Autodesk Inventor part; units mm, degrees
ref_plane "YZ Plane" through (0, 0, 0) normal (1, 0, 0) x (0, 1, 0)
ref_plane "XZ Plane" through (0, 0, 0) normal (0, 1, 0) x (-1, 0, 0)
ref_plane "XY Plane" through (0, 0, 0) normal (0, 0, 1) x (1, 0, 0)
sketch "Skizze1" plane through (0, 0, 0) normal (0, 0, 1) x (1, 0, 0)
  line L0 (46.5, 52.5) -> (-46.5, 52.5)
  line L1 (-46.5, 52.5) -> (-46.5, -52.5)
  line L2 (-46.5, -52.5) -> (46.5, -52.5)
  line L3 (46.5, -52.5) -> (46.5, 52.5)
  circle A0 centre (49, -60.25) radius 5.3
  circle A1 centre (49, -60.25) radius 2
  circle A2 centre (49, 60.25) radius 5.3
  circle A3 centre (49, 60.25) radius 2
  circle A4 centre (-61, 60.25) radius 5.3
  circle A5 centre (-61, 60.25) radius 2
  circle A6 centre (-61, -60.25) radius 5.3
  circle A7 centre (-61, -60.25) radius 2
  line L4 (49, 60.25) -> (-61, 60.25) construction
  line L5 (49, -60.25) -> (-61, -60.25) construction
  arc A8 (-59.9879, 65.4525) -> (47.9879, 65.4525) centre (-6, 342.9774) ccw
  arc A9 (47.9879, -65.4525) -> (-59.9879, -65.4525) centre (-6, -342.9774) ccw
  line L6 (-41.5, 39.5) -> (-41.5, -39.5)
  line L7 (41.5, -39.5) -> (41.5, 39.5)
  line L8 (38.5, 42.5) -> (-38.5, 42.5)
  line L9 (38.5, -42.5) -> (-38.5, -42.5)
  arc A10 (41.5, 39.5) -> (38.5, 42.5) centre (38.5, 39.5) ccw
  arc A11 (38.5, -42.5) -> (41.5, -39.5) centre (38.5, -39.5) ccw
  arc A12 (-41.5, -39.5) -> (-38.5, -42.5) centre (-38.5, -39.5) ccw
  arc A13 (-38.5, 42.5) -> (-41.5, 39.5) centre (-38.5, 39.5) ccw
  line L10 (-49, 42.5) -> (-49, -42.5)
  line L11 (49, 42.5) -> (49, -42.5)
  arc A14 (-64.7477, 56.5023) -> (-55.7, 51.2598) centre (-50.3799, 70.8701) ccw
  arc A15 (-49, 42.5) -> (-55.7, 51.2598) centre (-58.0765, 42.5) ccw
  arc A16 (-59.9879, 65.4525) -> (-64.7477, 56.5023) centre (-61, 60.25) ccw
  arc A17 (-55.7, -51.2598) -> (-64.7477, -56.5023) centre (-50.3799, -70.8701) ccw
  arc A18 (-55.7, -51.2598) -> (-49, -42.5) centre (-58.0765, -42.5) ccw
  arc A19 (-64.7477, -56.5023) -> (-59.9879, -65.4525) centre (-61, -60.25) ccw
  arc A20 (53.4323, 57.344) -> (49, 42.5) centre (76.0729, 42.5) ccw
  arc A21 (49, -42.5) -> (53.4323, -57.344) centre (76.0729, -42.5) ccw
  arc A22 (53.4323, 57.344) -> (47.9879, 65.4525) centre (49, 60.25) ccw
  arc A23 (47.9879, -65.4525) -> (53.4323, -57.344) centre (49, -60.25) ccw
  circle A24 centre (49, -60.25) radius 2.25
  circle A25 centre (-61, -60.25) radius 2.25
  circle A26 centre (-61, 60.25) radius 2.25
  circle A27 centre (49, 60.25) radius 2.25
  point P0 (-6, 60.25)
  point P1 (-6, -60.25)
  point P2 (-55.7, 60.25)
  dimension "d34" = 5
  dimension "d35" = 5
  dimension "d36" = 10
  dimension "d37" = 10
  dimension "d38" = 3
  dimension "d39" = 2.5
  dimension "d40" = 2.5
  dimension "d41" = 45
  dimension "d42" = 45
  dimension "d43" = 0.25
  dimension "d44" = 0.25
  dimension "d45" = 0.25
  dimension "d46" = 0.25
extrude "Extrusion1" add sketch "Skizze1" along normal blind 5 contours L3 L2 L1 L0 | A0 | A0 A9 A6 A17 A18 L10 A15 A14 A4 A8 A2 A20 L11 A21 | A6 | A2 | A4
sketch "Skizze2" plane through (0, 0, 0) normal (0, 0, -1) x (-1, 0, 0)
  arc A0 (59.9879, -65.4525) -> (64.7477, -56.5023) centre (61, -60.25) ccw
  arc A1 (64.7477, 56.5023) -> (59.9879, 65.4525) centre (61, 60.25) ccw
  line L0 (-46.5, 52.5) -> (46.5, 52.5)
  line L1 (46.5, 52.5) -> (46.5, -52.5)
  line L2 (46.5, -52.5) -> (-46.5, -52.5)
  line L3 (-46.5, -52.5) -> (-46.5, 52.5)
  line L4 (47, 53) -> (-47, 53)
  line L5 (-47, 53) -> (-47, -53)
  line L6 (-47, -53) -> (47, -53)
  line L7 (47, -53) -> (47, 53)
  arc A2 (-47.9879, 65.4525) -> (-53.4323, 57.344) centre (-49, 60.25) ccw
  arc A3 (-47.9879, 65.4525) -> (59.9879, 65.4525) centre (6, 342.9774) ccw
  arc A4 (-49, 42.5) -> (-53.4323, 57.344) centre (-76.0729, 42.5) ccw
  line L8 (-49, -42.5) -> (-49, 42.5)
  arc A5 (-53.4323, -57.344) -> (-49, -42.5) centre (-76.0729, -42.5) ccw
  arc A6 (-53.4323, -57.344) -> (-47.9879, -65.4525) centre (-49, -60.25) ccw
  arc A7 (59.9879, -65.4525) -> (-47.9879, -65.4525) centre (6, -342.9774) ccw
  arc A8 (64.7477, -56.5023) -> (55.7, -51.2598) centre (50.3799, -70.8701) ccw
  arc A9 (49, -42.5) -> (55.7, -51.2598) centre (58.0765, -42.5) ccw
  line L9 (49, 42.5) -> (49, -42.5)
  arc A10 (55.7, 51.2598) -> (49, 42.5) centre (58.0765, 42.5) ccw
  arc A11 (55.7, 51.2598) -> (64.7477, 56.5023) centre (50.3799, 70.8701) ccw
  circle A12 centre (61, 60.25) radius 2.25
  circle A13 centre (61, -60.25) radius 2.25
  circle A14 centre (-49, -60.25) radius 2.25
  circle A15 centre (-49, 60.25) radius 2.25
  point P0 (0, 0)
  dimension "d30" = 0.5
extrude "Extrusion2" add sketch "Skizze2" along normal blind 2 contours A7 A6 A5 L8 A4 A2 A3 A1 A11 A10 L9 A9 A8 A0 | L7 L6 L5 L4
equation "\"d35\" = d34"
equation "\"d37\" = d36"
equation "\"d40\" = d39"
equation "\"d44\" = d43"
equation "\"d45\" = d43"
equation "\"d46\" = d43"
properties part number "jetson_deckel"
For this review, take the finished solid that the model builds, in its own axes (mm). A direction names the side the tool comes from. Round coordinates to 2 decimals unless told otherwise and drop trailing zeros. Write each loop counter-clockwise with the first axis right and the second up, starting at its lowest first coordinate (ties: lowest second). Pieces come first, ordered by that corner, then holes. Notation, with made-up numbers: (26, 24.5) -> (68, 24.5) arc R25 ccw to (68, 46.5) -> close; hole circle Ø4 at (-4.75, 0.25). An arc over 180 degrees is marked (long way). Put each result on its own line as item: value.
Q1. Clearance check with flat-ended pins moving along their axes: pin 1 Ø0.6 at (x, z) = (17, -1.5) entering from -Y; pin 2 Ø1 at (y, z) = (-49, -1) entering from -X; pin 3 Ø1.5 at (y, z) = (-9, 3) entering from -X. State where each tip first meets the part, or that it passes through.
Determined:
pin 1: stops at y = -61.21
pin 2: stops at x = -52.3
pin 3: stops at x = -49
Q2. To check wall thickness, follow L1, parallel to X at y = 16.5, z = -1.5; L2, parallel to Y at x = -61, z = 3.95; L3, parallel to X at y = -19, z = 2.75. State the ranges of each line that lie inside material, in increasing order. Write a range as [from, to].
Determined:
L1: x = [-49, -46.5], [46.5, 49]
L2: y = [-65.55, -62.5], [-58, -53.55], [53.55, 58], [62.5, 65.55]
L3: x = [-49, -41.5], [41.5, 49]
Q3. Consider section B-B on x = 32.5. State the section outline as (y, z) points, and give its area (3 significant figures).
Determined:
outline: (-62.88, -2) -> (-52.5, -2) -> (-52.5, 0) -> (-42.5, 0) -> (-42.5, 5) -> (-62.88, 5) -> close; (42.5, 0) -> (52.5, 0) -> (52.5, -2) -> (62.88, -2) -> (62.88, 5) -> (42.5, 5) -> close
area: 245 mm^2
Q4. Consider section A-A on y = 22.5. State the section outline as (x, z) points, and give its area (3 significant figures).
Determined:
outline: (-49, -2) -> (-46.5, -2) -> (-46.5, 0) -> (-41.5, 0) -> (-41.5, 5) -> (-49, 5) -> close; (41.5, 0) -> (46.5, 0) -> (46.5, -2) -> (49, -2) -> (49, 5) -> (41.5, 5) -> close
area: 85.0 mm^2
Q5. The part is to be moulded in two halves that separate along X. For faces 5 (the cylindrical face through (50.163, 50.351, -0.986)), 6 (the cylindrical face through (-50.82, 47.95, -0.99)), 7 (the cylindrical face through (40.6, 41.64, 2.46)), 8 (the cylindrical face through (40.64, -41.6, 2.46)), say which applies: released by +X, released by -X, zero draft, split by the parting line, or undercut.
Determined:
face 5: released by +X
face 6: released by -X
face 7: undercut
face 8: undercut
Q6. Machinability: for faces 1 (the cylindrical face through (-40.64, 41.6, 2.46)), 2 (the cylindrical face through (-5.24, 60.25, 1.45)), 3 (the cylindrical face through (50.163, -50.351, 2.465)), 4 (the cylindrical face through (-60.5, -53.25, -0.99)), which of the approach directions +Z, -Z, +X, -X, +Y, -Y give a long, thin tool a straight path to every point of the face, cutting with its end or side? Answer none if there is none.
Determined:
face 1: +Z, -Z
face 2: +Z, -Z, +Y
face 3: +Z, -Z, +X
face 4: +Z, -Z, -X
Q7. Consider section C-C on z = 3.25. State the section outline as (x, y) points.
Determined:
outline: (-64.75, -56.5) arc R5.3 ccw to (-59.99, -65.45) arc R282.73 cw to (47.99, -65.45) arc R5.3 ccw to (53.43, -57.34) arc R27.07 cw to (49, -42.5) -> (49, 42.5) arc R27.07 cw to (53.43, 57.34) arc R5.3 ccw to (47.99, 65.45) arc R282.73 cw to (-59.99, 65.45) arc R5.3 ccw to (-64.75, 56.5) arc R20.32 ccw to (-55.7, 51.26) arc R9.08 cw to (-49, 42.5) -> (-49, -42.5) arc R9.08 cw to (-55.7, -51.26) arc R20.32 ccw to start; hole circle Ø4.5 at (-61, -60.25); hole circle Ø4.5 at (-61, 60.25); hole (-41.5, -39.5) arc R3 ccw to (-38.5, -42.5) -> (38.5, -42.5) arc R3 ccw to (41.5, -39.5) -> (41.5, 39.5) arc R3 ccw to (38.5, 42.5) -> (-38.5, 42.5) arc R3 ccw to (-41.5, 39.5) -> close; hole circle Ø4.5 at (49, -60.25); hole circle Ø4.5 at (49, 60.25)
